Can you work these out from the model? Positions are in its coordinate system, mm. Face numbers are marked on the shaded views. A direction names the side the tool comes from. Give positions to 0.01 mm unless a question says otherwise; leave off trailing zeros. Write each loop counter-clockwise with the first axis right and the second up, starting at its lowest first coordinate (ties: lowest second). Pieces come first, ordered by that corner, then holes. Notation, with made-up numbers: (68, 42.25) - (85, 42.25) arc R28 cw to (85, 66.25) - close; hole circle Ø10 at (80, 39). An arc over 180 degrees is marked (long way). Use a Markdown table: item, result. Add a question column.
```python
from build123d import *
from OCP.BRepAlgoAPI import BRepAlgoAPI_Cut
from OCP.TopTools import TopTools_ListOfShape

# Parameters (mm, degrees)
EXTRUDE_1_DEPTH          = 55
CUT_EXTRUDE_1_DEPTH      = 57.52709527297507
CUT_EXTRUDE_1_DEPTH_BACK = 57.52709527297507
SKETCH_2_W               = 2.5000000000000018
SKETCH_2_H               = 5.5000000000000036
SKETCH_2_H_2             = 5.499999999999993
SKETCH_2_H_3             = 5.5
CHAMFER_1_SIZE           = 2
SKETCH_3_R               = 1.8999999999999997
SKETCH_3_R_2             = 1.9000000000000001
CUT_EXTRUDE_2_DEPTH      = 57.52709527297507
SKETCH_4_R               = 4.025
CUT_EXTRUDE_3_DEPTH      = 2.5
CUT_EXTRUDE_4_DEPTH      = 3.8
EXTRUDE_START            = -1
EXTRUDE_2_DEPTH          = 1
FILLET_1_R               = 0.1


with BuildPart() as part:
    # 스케치1 → 보스-돌출1 (new body)
    with BuildSketch(Plane(origin=(0, 0, 0), x_dir=(1, 0, 0), z_dir=(0, 1, 0))):
        Polygon((-7.5, 0), (7.5, 0), (7.5, -2.5999999999999983), (10.5, -5.249999999999997), (8.000000000000002, -7.749999999999999), (-7.999999999999998, -7.750000000000001), (-10.5, -5.25), (-7.5, -2.6), align=None)
    extrude(amount=EXTRUDE_1_DEPTH)


with BuildPart() as cut_extrude_1_tool:
    # 스케치2 → 컷-돌출1 (new, two sides: drawn at the far end of the back side and taken through both)
    with BuildSketch(Plane(origin=(0, 0, 0), x_dir=(0, 0, -1), z_dir=(1, 0, 0)).offset(-CUT_EXTRUDE_1_DEPTH_BACK)):
        Polygon((-7.749999999999999, 4.549999999999999), (-5.249999999999997, 4.549999999999999), (-5.249999999999997, 10.049999999999997), (-7.749999999999999, 10.049999999999999), align=None)
        Polygon((-7.749999834765438, 20.150000000000002), (-5.249999834765436, 20.150000000000002), (-5.249999834765436, 14.649999999999999), (-7.749999834765438, 14.65), align=None)
        with Locations((-6.499999669530876, 27.5)):
            Rectangle(SKETCH_2_W, SKETCH_2_H)
        with Locations((-6.499999504296315, 37.599999999999994)):
            Rectangle(SKETCH_2_W, SKETCH_2_H_2)
        with Locations((-6.499999339061754, 47.699999999999996)):
            Rectangle(SKETCH_2_W, SKETCH_2_H_3)
    extrude(amount=CUT_EXTRUDE_1_DEPTH + CUT_EXTRUDE_1_DEPTH_BACK)


with BuildPart() as part_1:
    add(part.part)

    # 컷-돌출1: cut by cut_extrude_1_tool, with a tolerance
    cut_extrude_1_stock = TopTools_ListOfShape()
    cut_extrude_1_stock.Append(part_1.part.wrapped)
    cut_extrude_1_tools = TopTools_ListOfShape()
    cut_extrude_1_tools.Append(cut_extrude_1_tool.part.wrapped)
    cut_extrude_1_cut = BRepAlgoAPI_Cut()
    cut_extrude_1_cut.SetArguments(cut_extrude_1_stock)
    cut_extrude_1_cut.SetTools(cut_extrude_1_tools)
    cut_extrude_1_cut.SetFuzzyValue(0.00001)
    cut_extrude_1_cut.Build()
    add(Compound.cast(cut_extrude_1_cut.Shape()).solids(), mode=Mode.REPLACE)

    # 모따기1
    chamfer_1_edges = [part_1.edges().sort_by_distance(p)[0] for p in [
        (1.78e-15, 55, 7.75),
        (1.78e-15, 0, 7.75),
    ]]
    chamfer(chamfer_1_edges, length=CHAMFER_1_SIZE)

    # 스케치3 → 컷-돌출2 (cut, through all)
    with BuildSketch(Plane.XY):
        with Locations(Location((-3.47e-15, 47.699999999999996, 0), (0, 0, 180))):
            Circle(SKETCH_3_R)
        with Locations(Location((-3.47e-15, 7.299999999999997, 0), (0, 0, 180))):
            Circle(SKETCH_3_R_2)
    extrude(amount=CUT_EXTRUDE_2_DEPTH, mode=Mode.SUBTRACT)

    # 스케치4 → 컷-돌출3 (cut)
    with BuildSketch(Plane.XY.offset(7.75)):
        with Locations((-4.31e-15, 7.299999999999997)):
            Circle(SKETCH_4_R)
        with Locations((-4.31e-15, 47.699999999999996)):
            Circle(SKETCH_4_R)
    extrude(amount=-CUT_EXTRUDE_3_DEPTH, mode=Mode.SUBTRACT)

    # 모따기2
    # the kernel refuses this chamfer: 2, 1.738573476 mm, written as the material it takes off along each edge
    with BuildSketch(Plane(origin=(-3.47e-15, 47.699999999999996, 5.249999339061753), x_dir=(-1, 0, 0), z_dir=(0, -1, 0))) as chamfer_2_piece_1_section:
        with BuildLine():
            Line((3.9603767664178213, -0.05248472231924062), (1.839623233582178, 1.7910581979517))
            Line((1.839623233582178, 1.7910581979517), (1.799623233582178, 1.7910581979517))
            ThreePointArc((1.799623233582178, 1.7910581979517), (1.8599999999999997, 0.8955290989758504), (1.8599999999999997, 0))
            Line((1.8599999999999997, 0), (1.8999999999999997, -0.04000000000000004))
            ThreePointArc((1.8999999999999997, -0.04000000000000004), (2.9301883832089106, -0.04000000000000004), (3.9603767664178213, -0.09248472231924065))
            Line((3.9603767664178213, -0.09248472231924065), (3.9603767664178213, -0.05248472231924062))
        make_face()
    chamfer_2_piece_1 = revolve(axis=Axis((-3.47e-15, 47.699999999999996, 5.249999339061753), (0, 0, -1)), mode=Mode.PRIVATE)
    chamfer_2_piece_1 = split(chamfer_2_piece_1, bisect_by=Plane(origin=(-3.47e-15, 50.449999999999996, 5.249999339061753), z_dir=(0, -1, 0)), keep=Keep.TOP, mode=Mode.PRIVATE)
    chamfer_2_piece_1 = split(chamfer_2_piece_1, bisect_by=Plane(origin=(-3.47e-15, 44.949999999999996, 5.249999339061753), z_dir=(0, 1, 0)), keep=Keep.TOP, mode=Mode.PRIVATE)
    add(chamfer_2_piece_1, mode=Mode.SUBTRACT)
    with BuildSketch(Plane(origin=(-3.47e-15, 47.699999999999996, 5.249999339061753), x_dir=(-1, 0, 0), z_dir=(0, -1, 0))) as chamfer_2_piece_2_section:
        with BuildLine():
            Line((3.9603767664178213, -0.05248472231924062), (1.839623233582178, 1.7910581979517))
            Line((1.839623233582178, 1.7910581979517), (1.799623233582178, 1.7910581979517))
            ThreePointArc((1.799623233582178, 1.7910581979517), (1.8599999999999997, 0.8955290989758504), (1.8599999999999997, 0))
            Line((1.8599999999999997, 0), (1.8999999999999997, -0.04000000000000004))
            ThreePointArc((1.8999999999999997, -0.04000000000000004), (2.9301883832089106, -0.04000000000000004), (3.9603767664178213, -0.09248472231924065))
            Line((3.9603767664178213, -0.09248472231924065), (3.9603767664178213, -0.05248472231924062))
        make_face()
    chamfer_2_piece_2 = revolve(axis=Axis((-3.47e-15, 47.699999999999996, 5.249999339061753), (0, 0, -1)), mode=Mode.PRIVATE)
    chamfer_2_piece_2 = split(chamfer_2_piece_2, bisect_by=Plane(origin=(-3.47e-15, 44.949999999999996, 5.249999339061753), z_dir=(0, -1, 0)), keep=Keep.TOP, mode=Mode.PRIVATE)
    add(chamfer_2_piece_2, mode=Mode.SUBTRACT)
    with BuildSketch(Plane(origin=(-3.47e-15, 47.699999999999996, 5.249999339061753), x_dir=(-1, 0, 0), z_dir=(0, -1, 0))) as chamfer_2_piece_3_section:
        with BuildLine():
            Line((3.9603767664178213, -0.05248472231924062), (1.839623233582178, 1.7910581979517))
            Line((1.839623233582178, 1.7910581979517), (1.799623233582178, 1.7910581979517))
            ThreePointArc((1.799623233582178, 1.7910581979517), (1.8599999999999997, 0.8955290989758504), (1.8599999999999997, 0))
            Line((1.8599999999999997, 0), (1.8999999999999997, -0.04000000000000004))
            ThreePointArc((1.8999999999999997, -0.04000000000000004), (2.9301883832089106, -0.04000000000000004), (3.9603767664178213, -0.09248472231924065))
            Line((3.9603767664178213, -0.09248472231924065), (3.9603767664178213, -0.05248472231924062))
        make_face()
    chamfer_2_piece_3 = revolve(axis=Axis((-3.47e-15, 47.699999999999996, 5.249999339061753), (0, 0, -1)), mode=Mode.PRIVATE)
    chamfer_2_piece_3 = split(chamfer_2_piece_3, bisect_by=Plane(origin=(-3.47e-15, 50.449999999999996, 5.249999339061753), z_dir=(0, 1, 0)), keep=Keep.TOP, mode=Mode.PRIVATE)
    add(chamfer_2_piece_3, mode=Mode.SUBTRACT)
    with BuildSketch(Plane(origin=(-3.47e-15, 7.299999999999997, 5.249999999999997), x_dir=(-1, 0, 0), z_dir=(0, -1, 0))) as chamfer_2_piece_4:
        with BuildLine():
            Line((3.960376766417822, -0.05248472231924062), (1.8396232335821785, 1.7910581979517))
            Line((1.8396232335821785, 1.7910581979517), (1.7996232335821785, 1.7910581979517))
            ThreePointArc((1.7996232335821785, 1.7910581979517), (1.86, 0.8955290989758504), (1.86, 0))
            Line((1.86, 0), (1.9000000000000001, -0.04000000000000004))
            ThreePointArc((1.9000000000000001, -0.04000000000000004), (2.930188383208911, -0.04000000000000004), (3.960376766417822, -0.09248472231924065))
            Line((3.960376766417822, -0.09248472231924065), (3.960376766417822, -0.05248472231924062))
        make_face()
    revolve(axis=Axis((-3.47e-15, 7.299999999999997, 5.249999999999997), (0, 0, -1)), mode=Mode.SUBTRACT)

    # 스케치5 → 컷-돌출4 (cut)
    with BuildSketch(Plane.XY):
        with BuildLine():
            Line((2.95, 50.79999999999999), (2.9500000000000006, 47.699999999999996))
            ThreePointArc((2.9500000000000006, 47.699999999999996), (-4.01e-15, 44.75), (-2.9499999999999997, 47.699999999999996))
            Line((-2.9499999999999997, 47.699999999999996), (-2.95, 50.79999999999999))
            ThreePointArc((-2.95, 50.79999999999999), (1.7e-16, 53.74999999999999), (2.95, 50.79999999999999))
        make_face()
        with BuildLine():
            Line((-2.95, 7.299999999999997), (-2.95, 10.400000000000002))
            ThreePointArc((-2.95, 10.400000000000002), (1.8e-16, 13.350000000000001), (2.95, 10.400000000000002))
            Line((2.95, 10.400000000000002), (2.95, 7.299999999999997))
            ThreePointArc((2.95, 7.299999999999997), (-4.01e-15, 4.3500000000000005), (-2.95, 7.299999999999997))
        make_face()
    extrude(amount=CUT_EXTRUDE_4_DEPTH, mode=Mode.SUBTRACT)

    # 스케치6 → 보스-돌출2 (add)
    with BuildSketch(Plane.XY.offset(EXTRUDE_START)):
        with BuildLine():
            Line((-2.8696028673118352, 11.084017093292044), (-2.8696028673118352, 15.17002285126479))
            ThreePointArc((-2.8696028673118352, 15.17002285126479), (-2.97394354223574, 15.553533335617065), (-3.3160113650873604, 15.75591137943913))
            Line((-3.3160113650873604, 15.75591137943913), (-4.238447681040065, 15.894178508998346))
            ThreePointArc((-4.238447681040065, 15.894178508998346), (-4.485741808137749, 15.986176732767143), (-4.675, 16.17002285126479))
            ThreePointArc((-4.675, 16.17002285126479), (-3.3552259820417296, 19.565361197223766), (0, 20.984017093292046))
            ThreePointArc((0, 20.984017093292046), (3.355225982041729, 19.565361197223766), (4.675, 16.17002285126479))
            ThreePointArc((4.675, 16.17002285126479), (4.485741808137749, 15.986176732767143), (4.238447681040065, 15.894178508998346))
            Line((4.238447681040065, 15.894178508998346), (3.3160113650873604, 15.75591137943913))
            ThreePointArc((3.3160113650873604, 15.75591137943913), (2.9739435422357396, 15.553533335617065), (2.8696028673118352, 15.17002285126479))
            Line((2.8696028673118352, 15.17002285126479), (2.8696028673118352, 11.084017093292044))
            ThreePointArc((2.8696028673118352, 11.084017093292044), (1.8e-16, 13.350000000000001), (-2.8696028673118352, 11.084017093292044))
        make_face()
    extrude(amount=EXTRUDE_2_DEPTH)

    # 필렛1
    fillet_1_edges = [part_1.edges().sort_by_distance(p)[0] for p in [
        (-2.8696028673118352, 11.084017093292044, -0.5),
        (2.8696028673118352, 11.084017093292044, -0.5),
    ]]
    fillet(fillet_1_edges, radius=FILLET_1_R)


solid = part_1.part
```
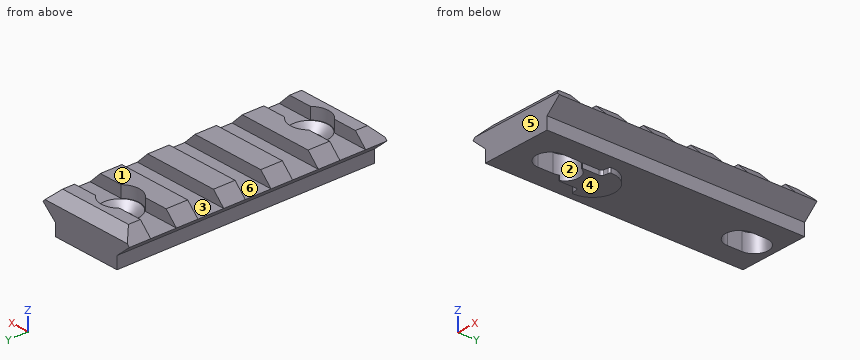
Q1. Suppose I cut it at B-B (x = 6.25). Please give me the cut outline in (y, z).
Q2. If I drill on probe 1 along Y at (x, z) = (-8.25, 5.75); probe 2 along Y at (x, z) = (3.25, 6); probe 3 along Y at (x, z) = (-2.5, 4.5), over which ranges is the centre line in solid material (lowest first)? Write a range as [from, to].
Q3. I'm going to push flat-ended pins straight in: P1, Ø2.5, axis at x = 4, y = 7, coming from the +Z side; P2, Ø0.8, axis at x = -6, z = 6.5, coming from the -Y side; P3, Ø0.8, axis at y = 36.5, z = 1, coming from the -X side. Where does each tip first touch, or does it pass through?
Q4. Suppose I cut it at C-C (x = 0.5). Give the number of separate pieces and of enclosed holes in the cut face, and give its area (3 significant figures).
Q5. Suppose I cut it at A-A (y = 24). Please give me the cut outline in (x, z).
Q6. On a 3-axis mill with a long thin cutter (end or side, diameter ignored), from which of +Z, -Z, +X, -X, +Y, -Y can I reach the whole of each face in a straight line? I mean the marked faces 1, 2 and 3. Say none if no direction works.
Q7. If we mould it in two halves opening along Y, with no side actions, what happens to the marked faces 4, 5 and 6? For each: released by +Y, released by -Y, zero draft, split by the parting line, or undercut.
Derived:
| question | item | result |
|---|---|---|
| 1 | outline | (0, 0) - (55, 0) - (55, 5.75) - (53, 7.75) - (50.45, 7.75) - (50.45, 5.25) - (44.95, 5.25) - (44.95, 7.75) - (40.35, 7.75) - (40.35, 5.25) - (34.85, 5.25) - (34.85, 7.75) - (30.25, 7.75) - (30.25, 5.25) - (24.75, 5.25) - (24.75, 7.75) - (20.15, 7.75) - (20.15, 5.25) - (14.65, 5.25) - (14.65, 7.75) - (10.05, 7.75) - (10.05, 5.25) - (4.55, 5.25) - (4.55, 7.75) - (2, 7.75) - (0, 5.75) - close |
| 2 | probe 1 | [0, 4.55], [10.05, 14.65], [20.15, 24.75], [30.25, 34.85], [40.35, 44.95], [50.45, 55] |
| 2 | probe 2 | [0.25, 4.55], [10.05, 14.65], [20.15, 24.75], [30.25, 34.85], [40.35, 44.95], [50.45, 54.75] |
| 2 | probe 3 | [0, 5.58], [9.02, 45.98], [49.42, 55] |
| 3 | P1 | z = 5.25 |
| 3 | P2 | y = 0.35 |
| 3 | P3 | x = -7.5 |
| 4 | separate pieces | 3 |
| 4 | enclosed holes | 0 |
| 4 | area | 263 mm² |
| 5 | outline | (-10.5, 5.25) - (-7.5, 2.6) - (-7.5, 0) - (7.5, 0) - (7.5, 2.6) - (10.5, 5.25) - (8, 7.75) - (-8, 7.75) - close |
| 6 | face 1 | +Z, +X, -X, +Y, -Y |
| 6 | face 2 | -Z |
| 6 | face 3 | +Z, +X, -X |
| 7 | face 4 | zero draft |
| 7 | face 5 | released by -Y |
| 7 | face 6 | undercut |
